For this review, take the finished solid that the model builds, in its own axes (mm). A direction names the side the tool comes from. Give positions to 0.01 mm unless a question says otherwise; leave off trailing zeros. Write each loop counter-clockwise with the first axis right and the second up, starting at its lowest first coordinate (ties: lowest second). Pieces come first, ordered by that corner, then holes. Notation, with made-up numbers: M 9,81.5 L 52,81.5 A25 ccw 52,98.5 Z; hole C 76.25,6 d8. An arc over 180 degrees is marked long. One line per item, written item: value. Start each with the question number.
Item 1: Consider section C-C, the plane y = 13.75. Write out the cut boundary in (x, z).
Item 2: Mouldability with a two-part tool opening along Y and no side actions: class faces 5 (the face through (14, 0, 0)), 6 (the face through (3.9, 1, -1)), 7 (the face through (14, 25.8, 2)), 8 (the face through (4.306, 22.635, -0.246)) as released by +Y, released by -Y, zero draft, split by the parting line, or undercut.
Item 3: Tool access review of faces 1 (the face through (24.105, 22.413, -0.246)), 2 (the face through (5, 24, 2)), 3 (the face through (14, 18.55, 2)), 4 (the face through (25, 25, -0.5)): name each direction out of +Z, -Z, +X, -X, +Y, -Y from which nothing blocks a thin tool from reaching the whole face with its end or side.
Item 4: Consider section D-D, the plane x = 21.25. Write out the cut boundary in (y, z), and give its area (3 significant figures).
Item 5: To check wall thickness, follow probe 1 along X at (y, z) = (11.61, 1.3); probe 2 along X at (y, z) = (23.9, 1); probe 3 along Y at (x, z) = (3.5, 2.75) (3 decimals). State the ranges of each line that lie inside material, in increasing order.
Item 6: Consider section A-A, the plane y = 23.9. Give the number of separate pieces and of enclosed holes in the cut face, and give its area (3 significant figures).
Item 7: Clearance check with flat-ended pins moving along their axes: pin 1 Ø1.5 at (x, z) = (3.5, -1) entering from +Y; pin 2 Ø2.5 at (x, y) = (24.3, 23.9) entering from +Z; pin 3 Ø1 at (x, y) = (6.5, 8.5) entering from -Z. State where each tip first meets the part, or that it passes through.
Item 8: Consider section B-B, the plane x = 3.5. Write out the cut boundary in (y, z) (3 decimals), and give its area (3 significant figures).
```python
from build123d import *

# Parameters (mm, degrees)
SKETCH_W        = 27.8
SKETCH_H        = 25.8
SKETCH_R        = 1
SKETCH_W_2      = 12.8
SKETCH_H_2      = 11.05
PAD_DEPTH       = 3
SKETCH002_W     = 20
SKETCH002_H     = 2
PAD001_DEPTH    = 2
SKETCH003_R     = 1.5
SKETCH003_R_2   = 1
PAD002_DEPTH    = 0.5
SKETCH005_R     = 1.75
POCKET_DEPTH    = 1
SKETCH006_W     = 8
SKETCH006_H     = 7.25
POCKET001_DEPTH = 1.5


with BuildPart() as part:
    # Sketch → Pad (new body)
    with BuildSketch(Plane.XY):
        with Locations((13.9, 12.9)):
            Rectangle(SKETCH_W, SKETCH_H)
        with Locations((3.5, 23.9)):
            Circle(SKETCH_R, mode=Mode.SUBTRACT)
        with Locations((24.3, 23.9)):
            Circle(SKETCH_R, mode=Mode.SUBTRACT)
        with Locations((23.95, 11.61)):
            Circle(SKETCH_R, mode=Mode.SUBTRACT)
        with Locations((3.5, 11.545)):
            Circle(SKETCH_R, mode=Mode.SUBTRACT)
        with Locations((13.9, 13.025)):
            Rectangle(SKETCH_W_2, SKETCH_H_2, mode=Mode.SUBTRACT)
    extrude(amount=PAD_DEPTH)

    # Sketch002 → Pad001 (join)
    with BuildSketch(Plane.XY):
        with Locations((13.9, 1)):
            Rectangle(SKETCH002_W, SKETCH002_H)
    extrude(amount=-PAD001_DEPTH)

    # Sketch003 (on Face13 of Pad) → Pad002 (join)
    with BuildSketch(Plane(origin=(0, 0, 0), x_dir=(1, 0, 0), z_dir=(0, 0, -1))):
        with Locations((24.3, -23.9)):
            Circle(SKETCH003_R)
        with Locations((24.3, -23.9)):
            Circle(SKETCH003_R_2, mode=Mode.SUBTRACT)
        with Locations((3.5, -23.9)):
            Circle(SKETCH003_R)
        with Locations((3.5, -23.9)):
            Circle(SKETCH003_R_2, mode=Mode.SUBTRACT)
        with Locations((23.95, -11.61)):
            Circle(SKETCH003_R)
        with Locations((23.95, -11.61)):
            Circle(SKETCH003_R_2, mode=Mode.SUBTRACT)
        with Locations((3.5, -11.545)):
            Circle(SKETCH003_R)
        with Locations((3.5, -11.545)):
            Circle(SKETCH003_R_2, mode=Mode.SUBTRACT)
    extrude(amount=PAD002_DEPTH)

    # Sketch005 (on Face6 of Pad002) → Pocket (cut)
    with BuildSketch(Plane.XY.offset(3)):
        with Locations((23.95, 11.61)):
            Circle(SKETCH005_R)
        with Locations((3.5, 11.545)):
            Circle(SKETCH005_R)
        with Locations((3.5, 23.9)):
            Circle(SKETCH005_R)
        with Locations((24.3, 23.9)):
            Circle(SKETCH005_R)
    extrude(amount=-POCKET_DEPTH, mode=Mode.SUBTRACT)

    # Sketch006 (on Face4 of Pad001) → Pocket001 (cut)
    with BuildSketch(Plane(origin=(0, 0, 0), x_dir=(1, 0, 0), z_dir=(0, 0, -1))):
        with Locations((13.9, -22.175)):
            Rectangle(SKETCH006_W, SKETCH006_H)
    extrude(amount=-POCKET001_DEPTH, mode=Mode.SUBTRACT)


solid = part.part
```
Model answer:
1. outline: M 0,0 L 7.5,0 L 7.5,3 L 0,3 Z; M 20.3,0 L 27.8,0 L 27.8,3 L 20.3,3 Z
2. face 5: released by -Y
2. face 6: zero draft
2. face 7: released by +Y
2. face 8: undercut
3. face 1: -Z
3. face 2: +Z
3. face 3: +Z, -Z
3. face 4: -Z, +X, -X, +Y
4. outline: M 0,-2 L 2,-2 L 2,0 L 25.8,0 L 25.8,3 L 0,3 Z
4. area: 81.4 mm2
5. probe 1: x = 0 to 2.5, 4.5 to 7.5, 20.3 to 22.95, 24.95 to 27.8
5. probe 2: x = 0 to 2.5, 4.5 to 9.9, 17.9 to 23.3, 25.3 to 27.8
5. probe 3: y = 0 to 9.795, 13.295 to 22.15, 25.65 to 25.8
6. separate pieces: 3
6. enclosed holes: 0
6. area: 57.4 mm2
7. pin 1: stops at y = 25.4
7. pin 2: stops at z = 2
7. pin 3: stops at z = 0
8. outline: M 0,0 L 10.045,0 L 10.045,-0.5 L 10.545,-0.5 L 10.545,2 L 9.795,2 L 9.795,3 L 0,3 Z; M 12.545,-0.5 L 13.045,-0.5 L 13.045,0 L 22.4,0 L 22.4,-0.5 L 22.9,-0.5 L 22.9,2 L 22.15,2 L 22.15,3 L 13.295,3 L 13.295,2 L 12.545,2 Z; M 24.9,-0.5 L 25.4,-0.5 L 25.4,0 L 25.8,0 L 25.8,3 L 25.65,3 L 25.65,2 L 24.9,2 Z
8. area: 63.4 mm2
